Verification items for the finished model (mm, model axes). A direction names the side the tool comes from. Round coordinates to 2 decimals unless told otherwise and drop trailing zeros. Order: outer loops, then holes, each group sorted by start corner. A loop starts at its lowest first (then second) coordinate and runs counter-clockwise, first axis right, second up. Notation, with made-up numbers: (74, 7.5) -> (105, 7.5) arc R24 cw to (105, 44.5) -> close; hole circle Ø3 at (-25.5, 76). An arc over 180 degrees is marked (long way). Return JSON: item names as keys, results as strings. Group by question number.
1) Depth check by flat-ended pin: pin 1 (1.8 mm diameter, centred on x = -2, z = 0.5, fed in from -Y); pin 2 (1.1 mm diameter, centred on x = -2, z = 0.5, fed in from +Y); pin 3 (5 mm diameter, centred on x = 3.5, z = 0, fed in from -Y). Enter the tip coordinate at first touch or a pass-through.
2) Tool access check on faces 4 (the flat face through (8, 0, 0)), 5 (the flat face through (0, 0, 4)), 6 (the flat face through (-2.19, -0.99, 1.74)). Record the directions out of +Z, -Z, +X, -X, +Y, -Y that give a thin tool (end or side, any length) a straight path to the whole face; none if there is none.
3) Section check A-A on x = 2.25. Enter the section's corners in (y, z), plus the area to 3 significant figures.
4) Scan lines: L1, parallel to X at y = 1.5, z = -4.25; L2, parallel to X at y = 3.75, z = -2.75; L3, parallel to Y at x = 2.75, z = 1. Record each from-to range of solid material in increasing order.
5) Draft check along Y on faces 1 (the flat face through (-2, -2, 0)), 2 (the cylindrical face through (-0.4, 5, -1.6)), 3 (the flat face through (-3.3, 1, 2)). Enter one of: pulls with the +Y half, pulls with the -Y half, needs draft (parallel to the pull), parting line crosses it, or undercut.
Autodesk Inventor part; units mm, degrees
ref_plane "Work Plane1" through (29, 0, 0) normal (0, -1, 0) x (1, 0, 0)
ref_plane "YZ Plane" through (0, 0, 0) normal (1, 0, 0) x (0, 1, 0)
ref_plane "XZ Plane" through (0, 0, 0) normal (0, 1, 0) x (-1, 0, 0)
sketch "Sketch1" plane through (0, 0, 0) normal (0, 0, 1) x (1, 0, 0)
  line L0 (0.1133, 0) -> (8, 0)
  line L1 (8, 0) -> (8, 3)
  line L2 (8, 3) -> (1, 3)
  line L3 (1, 3) -> (0.3865, 3)
  line L4 (0.3865, 3) -> (0, 3)
  line L5 (0, 3) -> (0, 5.25)
  line L6 (0, 5.25) -> (-3.3, 5.25)
  line L7 (-3.3, 5.25) -> (-3.3, 2.3094)
  line L8 (-3.3, 2.3094) -> (-1.22, 2.3094)
  line L9 (-1.22, 2.3094) -> (0.1133, 0)
  line L10 (-5.56, 0) -> (10.26, 0)
  line L11 (0, -1.05) -> (0, 6.3)
  line L12 (1, 3) -> (0, 3) construction
  dimension "d1" = 7
  dimension "d2" = 0.6136
  dimension "d3" = 3.3
  dimension "d4" = 2.08
  dimension "d5" = 60
  dimension "d6" = 6
  dimension "d7" = 6
  dimension "d8" = 4.6188
  dimension "d9" = 10.5
  dimension "d26" = 8
revolve "Body" add sketch "Sketch1" angle 360 about axis through (0.1133, 0, 0) along (1, 0, 0) contours L9 L11 L4 L3 L2 L1 L0 | L9 L8 L7 L6 L5 L11
sketch "Sketch2" plane through (-3.3, 0, 0) normal (-1, 0, 0) x (0, 0, 1)
  circle A0 centre (0, 0) radius 2.3094
  line L0 (0, -7.35) -> (0, 7.35)
  line L1 (-7.35, 0) -> (7.35, 0)
  line L2 (2.3094, 0) -> (1.1547, -2)
  line L3 (1.1547, -2) -> (-1.1547, -2)
  line L4 (-1.1547, -2) -> (-2.3094, 0)
  line L5 (-2.3094, 0) -> (-1.1547, 2)
  line L6 (-1.1547, 2) -> (1.1547, 2)
  line L7 (1.1547, 2) -> (2.3094, 0)
extrude "Slot" add sketch "Sketch2" against normal up to next contours L7 A0 | A0 L2 | L6 L0 A0 | A0 L0 L3 | L0 L6 A0 | A0 L3 L0 | L4 A0 | A0 L5
fillet "Fillet1" radius 2.56 1 edges at (-3.3, -5.25, 0)
thread "Thread"
chamfer "Chamfer1" distance 0.6135 distance2 0.6135 1 edges at (8, -3, 0) measured on face at (8, 0.705, 0.3049)
ref_plane "Work Plane1" through (29, 0, 0) normal (0, -1, 0) x (1, 0, 0)
fillet "Fillet2" radius 0.5 1 edges at (0, -3, 0)
equation "\"d30\" = R"
equation "\"d17\" = RR"
equation "\"d13\" = GEL"
equation "\"d15\" = -0.5 * SPD + 0.5 * GD"
equation "\"d16\" = GUL"
equation "\"d1\" = GEL"
equation "\"d3\" = KOH"
equation "\"d4\" = INTI"
equation "\"d6\" = GD"
equation "\"d7\" = BDM"
equation "\"d8\" = 1.1547 * SW"
equation "\"d9\" = KOD"
equation "\"GD\" = NND"
equation "\"GEL\" = 7"
equation "\"KOD\" = 10.5"
equation "\"KOH\" = 3.3"
equation "\"INTI\" = 2.08"
equation "\"GAL\" = 0.61345 * PTC"
equation "\"GUL\" = 0.61345 * PTC"
equation "\"BDM\" = NND"
equation "\"SW\" = 4"
equation "\"RR\" = 2.56"
equation "\"SPD\" = NND - 1.2269 * PTC"
equation "\"R\" = 0.5"
equation "\"TOA\" = 30deg"
equation "\"GD1\" = THREADDIA - 1.2269 * PTC"
equation "\"THREADDIA\" = 6"
equation "\"PTC\" = 1"
equation "\"NND\" = 6"
equation "\"KOH1\" = 0.74"
equation "\"E0\" = 4.583"
properties part number "ISO 7380-1 - M6 x 10" material "Steel"
Check result:
{
 "1": {"pin 1": "y = -5.21", "pin 2": "y = 5.13", "pin 3": "y = -3"},
 "2": {"face 4": "+Z, -Z, +X, +Y, -Y", "face 5": "+X", "face 6": "-X"},
 "3": {"outline": "circle Ø6 at (0, 0)", "area": "28.3 mm^2"},
 "4": {"L1": "-2.54 to 0", "L2": "-2.39 to 0", "L3": "-2.83 to 2.83"},
 "5": {"face 1": "undercut", "face 2": "parting line crosses it", "face 3": "needs draft"}
}
